from build123d import *

# Parameters (mm, degrees)
EXTRUSION1_DEPTH = 10
ESQUISSE2_R      = 1.5
EXTRUSION2_DEPTH = 18


with BuildPart() as part:
    # Esquisse1 → Extrusion1 (new body)
    with BuildSketch(Plane.XY):
        with BuildLine():
            Line((17.773719933, 3), (-17.773719933, 3))
            Line((-17.773719933, 3), (-19.446474381, 4.672754448))
            ThreePointArc((-19.446474381, 4.672754448), (0, 20), (19.446474381, 4.672754448))
            Line((19.446474381, 4.672754448), (17.773719933, 3))
        make_face()
    extrude(amount=EXTRUSION1_DEPTH)

    # Esquisse2 → Extrusion2 (cut, through all)
    with BuildSketch(Plane.XZ.offset(-3)):
        with Locations((-12, 3)):
            Circle(ESQUISSE2_R)
        with Locations((12, 3)):
            Circle(ESQUISSE2_R)
    extrude(amount=-EXTRUSION2_DEPTH, mode=Mode.SUBTRACT)


solid = part.part
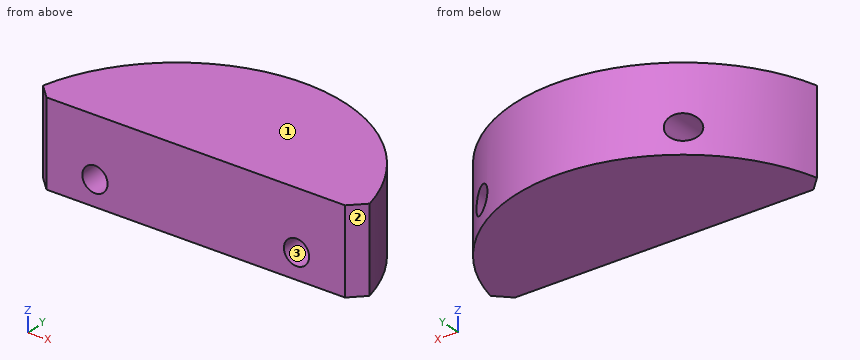
Geometry: final body of the model. Coordinates: model frame, mm. Face numbers are marked on the shaded views. Give positions to 0.01 mm unless a question says otherwise; leave off trailing zeros. Write each loop counter-clockwise with the first axis right and the second up, starting at its lowest first coordinate (ties: lowest second). Pieces come first, ordered by that corner, then holes. Notation, with made-up numbers: M 75.5,-1.75 L 125.5,-1.75 A16 ccw 125.5,27.25 Z; hole C 0,20.5 d2. An arc over 180 degrees is marked long. Answer in a Markdown table with one row per item. Add a question column.
(1) First-contact query: pin 1 (2 mm diameter, centred on x = 15.5, z = 1.5, fed in from +Y) (3 decimals); pin 2 (1 mm diameter, centred on y = 10, z = 7.5, fed in from +X); pin 3 (5 mm diameter, centred on x = -12, z = 3, fed in from +Y). Flat tips, straight axial feed; report the tip coordinate or a pass-through.
(2) Ray query, line 1 (Z direction, x = -12, y = 6.75); line 2 (X direction, y = 12.75, z = 3); line 3 (X direction, y = 5.5, z = 2). Return the intervals inside material, ascending.
(3) Mould query, pull axis Z, two halves, no side actions, for the marked faces 1, 2 and 3. Classes: +Z half, -Z half, draft (parallel to the pull), parting line (faces both ways), or undercut.
(4) Section D-D on z = 5.25. Return loops of the section in (x, y), and give its area (3 significant figures).
(5) Section A-A on x = 12. Return loops of the section in (y, z).
(6) Section B-B on z = 3. Return loops of the section in (x, y), and give its area (3 significant figures).
(7) Section C-C on y = 16. Return loops of the section in (x, z).
Result set:
| question | item | result |
|---|---|---|
| 1 | pin 1 | stops at y = 13.775 |
| 1 | pin 2 | stops at x = 17.6 |
| 1 | pin 3 | stops at y = 17.6 |
| 2 | line 1 | z = 0 to 1.5, 4.5 to 10 |
| 2 | line 2 | x = -15.41 to -13.5, -10.5 to 10.5, 13.5 to 15.41 |
| 2 | line 3 | x = -19.23 to -13.12, -10.88 to 10.88, 13.12 to 19.23 |
| 3 | face 1 | +Z half |
| 3 | face 2 | draft |
| 3 | face 3 | undercut |
| 4 | outline | M -19.45,4.67 L -17.77,3 L 17.77,3 L 19.45,4.67 A20 ccw Z |
| 4 | area | 505 mm^2 |
| 5 | outline | M 3,0 L 16,0 L 16,1.5 L 3,1.5 Z; M 3,4.5 L 16,4.5 L 16,10 L 3,10 Z |
| 6 | outline | M -19.45,4.67 L -17.77,3 L -13.5,3 L -13.5,14.76 A20 ccw Z; M -10.5,3 L 10.5,3 L 10.5,17.02 A20 ccw -10.5,17.02 Z; M 13.5,3 L 17.77,3 L 19.45,4.67 A20 ccw 13.5,14.76 Z |
| 6 | area | 428 mm^2 |
| 7 | outline | M -12,0 L 12,0 L 12,1.5 A1.5 cw 12,4.5 L 12,10 L -12,10 L -12,4.5 A1.5 cw -12,1.5 Z |
